Part model, mm, in its own coordinate system. A direction names the side the tool comes from. Round coordinates to 2 decimals unless told otherwise and drop trailing zeros. Write each loop counter-clockwise with the first axis right and the second up, starting at its lowest first coordinate (ties: lowest second). Pieces come first, ordered by that corner, then holes. Notation, with made-up numbers: M 43,57.5 L 59,57.5 A33 ccw 59,95.5 Z; hole C -5.75,55.25 d11. An arc over 180 degrees is marked long. Answer as a JSON object with one key per item and string values. Group by question number.
1. Drop flat-ended pins along their axis: pin 1 (9 mm diameter, centred on x = 0, y = 313.5, fed in from +Z); pin 2 (7 mm diameter, centred on x = 154.5, y = -5, fed in from -Z). Give the stop position or say it passes through.
2. Band-saw the part on A-A, the plane x = -23. Write the cut outline in (y, z), plus the area to 3 significant figures.
3. Drill centre lines: line 1 (Y direction, x = 0, z = 4); line 2 (Y direction, x = 120, z = -2.5); line 3 (Y direction, x = 128, z = -2.75). Where is each one in solid material? Low to high. Write a range as from..to.
4. Band-saw the part on B-B, the plane y = 104.5. Write the cut outline in (x, z), plus the area to 3 significant figures.
5. Two-plate mould, pull along X, no slides. Class faces 3 (the face through (3, -16.5, 0)), 4 (the face through (-187.15, 12.51, 0.11)), 5 (the face through (219, 152, 0)): +X half, -X half, draft (parallel to the pull), parting line (faces both ways), or undercut.
6. Which spindle directions (+Z, -Z, +X, -X, +Y, -Y) get a long thin tool onto all of the face, cutting with end or side? Do faces 1 (the face through (-54.547, -4.041, -4.194)), 2 (the face through (174.64, 113.04, 0.11)). Say none if no direction does.
from build123d import *
from build123d.topology import SkipClean

# Parameters (mm, degrees)
ESQUISSE1_R        = 3
ESQUISSE1_R_2      = 3.5
BOSS_EXTRU_1_DEPTH = 8
CHANFREIN1_SIZE    = 4


with BuildPart() as part:
    # Esquisse1 → Boss.-Extru.1 (new body, symmetric)
    with BuildSketch(Plane.XY):
        with BuildLine():
            Line((0, 9.5), (0, -2))
            ThreePointArc((0, -2), (3, -5), (0, -8))
            Line((0, -8), (0, -16.5))
            Line((0, -16.5), (219, -16.5))
            Line((219, -16.5), (219, 325))
            Line((219, 325), (0, 325))
            Line((0, 325), (0, 317))
            ThreePointArc((0, 317), (3.5, 313.5), (0, 310))
            Line((0, 310), (0, 162))
            ThreePointArc((0, 162), (3.5, 158.5), (0, 155))
            Line((0, 155), (0, 135))
            Line((0, 135), (154.64816242, 135))
            ThreePointArc((154.64816242, 135), (159.366741675, 133.816745988), (162.968665363, 130.547001962))
            Line((162.968665363, 130.547001962), (186.641005887, 95.03849117))
            ThreePointArc((186.641005887, 95.03849117), (189.14184053, 89.740170219), (190, 83.944487245))
            Line((190, 83.944487245), (190, 19.5))
            ThreePointArc((190, 19.5), (187.071067812, 12.428932188), (180, 9.5))
            Line((180, 9.5), (0, 9.5))
        make_face()
        with Locations((188, 278)):
            Circle(ESQUISSE1_R, mode=Mode.SUBTRACT)
        with Locations((158, 278)):
            Circle(ESQUISSE1_R, mode=Mode.SUBTRACT)
        with Locations((128, 278)):
            Circle(ESQUISSE1_R, mode=Mode.SUBTRACT)
        with Locations((51.5, -5)):
            Circle(ESQUISSE1_R, mode=Mode.SUBTRACT)
        with Locations((103, -5)):
            Circle(ESQUISSE1_R, mode=Mode.SUBTRACT)
        with Locations((154.5, -5)):
            Circle(ESQUISSE1_R, mode=Mode.SUBTRACT)
        with Locations((206, -5)):
            Circle(ESQUISSE1_R, mode=Mode.SUBTRACT)
        with Locations((128, 194)):
            Circle(ESQUISSE1_R, mode=Mode.SUBTRACT)
        with Locations((158, 194)):
            Circle(ESQUISSE1_R, mode=Mode.SUBTRACT)
        with Locations((188, 194)):
            Circle(ESQUISSE1_R, mode=Mode.SUBTRACT)
        with Locations((211, 268)):
            Circle(ESQUISSE1_R, mode=Mode.SUBTRACT)
        with Locations((211, 130)):
            Circle(ESQUISSE1_R, mode=Mode.SUBTRACT)
        with Locations((211, 93)):
            Circle(ESQUISSE1_R, mode=Mode.SUBTRACT)
        with Locations((211, 170.5)):
            Circle(ESQUISSE1_R, mode=Mode.SUBTRACT)
        with Locations((211, 315)):
            Circle(ESQUISSE1_R, mode=Mode.SUBTRACT)
        with Locations((211, 56)):
            Circle(ESQUISSE1_R, mode=Mode.SUBTRACT)
        with Locations((211, 19)):
            Circle(ESQUISSE1_R, mode=Mode.SUBTRACT)
        with Locations((211, 204)):
            Circle(ESQUISSE1_R, mode=Mode.SUBTRACT)
        with Locations((60, 158.5)):
            Circle(ESQUISSE1_R_2, mode=Mode.SUBTRACT)
        with Locations((120, 158.5)):
            Circle(ESQUISSE1_R_2, mode=Mode.SUBTRACT)
        with Locations((180, 158.5)):
            Circle(ESQUISSE1_R_2, mode=Mode.SUBTRACT)
        with Locations((180, 313.5)):
            Circle(ESQUISSE1_R_2, mode=Mode.SUBTRACT)
        with Locations((60, 313.5)):
            Circle(ESQUISSE1_R_2, mode=Mode.SUBTRACT)
        with Locations((120, 313.5)):
            Circle(ESQUISSE1_R_2, mode=Mode.SUBTRACT)
    boss_extru_1 = extrude(amount=BOSS_EXTRU_1_DEPTH, both=True)

    # Sym_trie1: Boss.-Extru.1 across plane
    with SkipClean():  # keep this step's faces unmerged: merging them makes the solid invalid here
        add(boss_extru_1.mirror(Plane(origin=(0, 0, 0), x_dir=(0, 0, 1), z_dir=(1, 0, 0))))

    # Chanfrein1
    chanfrein1_edges = [part.edges().sort_by_distance(p)[0] for p in [
        (-48.5, -5, -8),
        (-100, -5, -8),
        (-151.5, -5, -8),
        (-203, -5, -8),
        (3, -5, -8),
        (48.5, -5, -8),
        (100, -5, -8),
        (151.5, -5, -8),
        (203, -5, -8),
    ]]
    chamfer(chanfrein1_edges, length=CHANFREIN1_SIZE)


solid = part.part
Worked answers:
{
 "1": {"pin 1": "stops at z = 8", "pin 2": "stops at z = -4.5"},
 "2": {"outline": "M -16.5,-8 L 9.5,-8 L 9.5,8 L -16.5,8 Z; M 135,-8 L 325,-8 L 325,8 L 135,8 Z", "area": "3,460 mm^2"},
 "3": {"line 1": "y = -16.5..-8, -2..9.5, 135..155, 162..310, 317..325", "line 2": "y = -16.5..9.5, 135..155, 162..310, 317..325", "line 3": "y = -16.5..9.5, 135..191, 197..275, 281..325"},
 "4": {"outline": "M -219,-8 L -180.33,-8 L -180.33,8 L -219,8 Z; M 180.33,-8 L 219,-8 L 219,8 L 180.33,8 Z", "area": "1,240 mm^2"},
 "5": {"face 3": "draft", "face 4": "undercut", "face 5": "+X half"},
 "6": {"face 1": "-Z", "face 2": "+Z, -Z"}
}
